The figure shows three views and two pictorial views of one solid part (mm, origin at its lowest corner). Answer the questions. Coordinates: 2 decimals unless noted, no trailing zeros. Write each loop counter-clockwise with the first axis right and the second up, starting at its lowest first coordinate (ties: lowest second). Pieces come first, ordered by that corner, then holes.
Item 1: Straight lines are drawn through the part: probe 1 along Y at (x, z) = (12.75, 141.5) (1 decimal); probe 2 along X at (y, z) = (15.5, 110); probe 3 along X at (y, z) = (5.5, 56.5) (1 decimal). For each, find the intervals that lie inside material, in ascending order.
Item 2: Section C-C (y = 18.5) is taken. Give the vertices of the cut face in (x, z) (1 decimal).
Item 3: Each of these flat-tipped pins is pushed along its axis until it touches: P1, Ø8, axis at x = 4, z = 95.5, coming from the -Y side; P2, Ø10, axis at y = 29.5, z = 152.5, coming from the +X side; P3, Ø3, axis at x = 1.5, z = 200, coming from the -Y side (1 decimal); P4, Ø1.9, axis at x = 4, z = 201.5, coming from the +Y side (1 decimal). Where does it stop, or does it pass through?
Item 4: Determine the mould class of the marked faces 1, 2, 3 and 4 for opening direction Y: released by +Y, released by -Y, zero draft, split by the parting line, or undercut.
Item 5: Section A-A (x = 10.5) is taken. Give the vertices of the cut face in (y, z) (1 decimal), then the cut area to 3 significant figures.
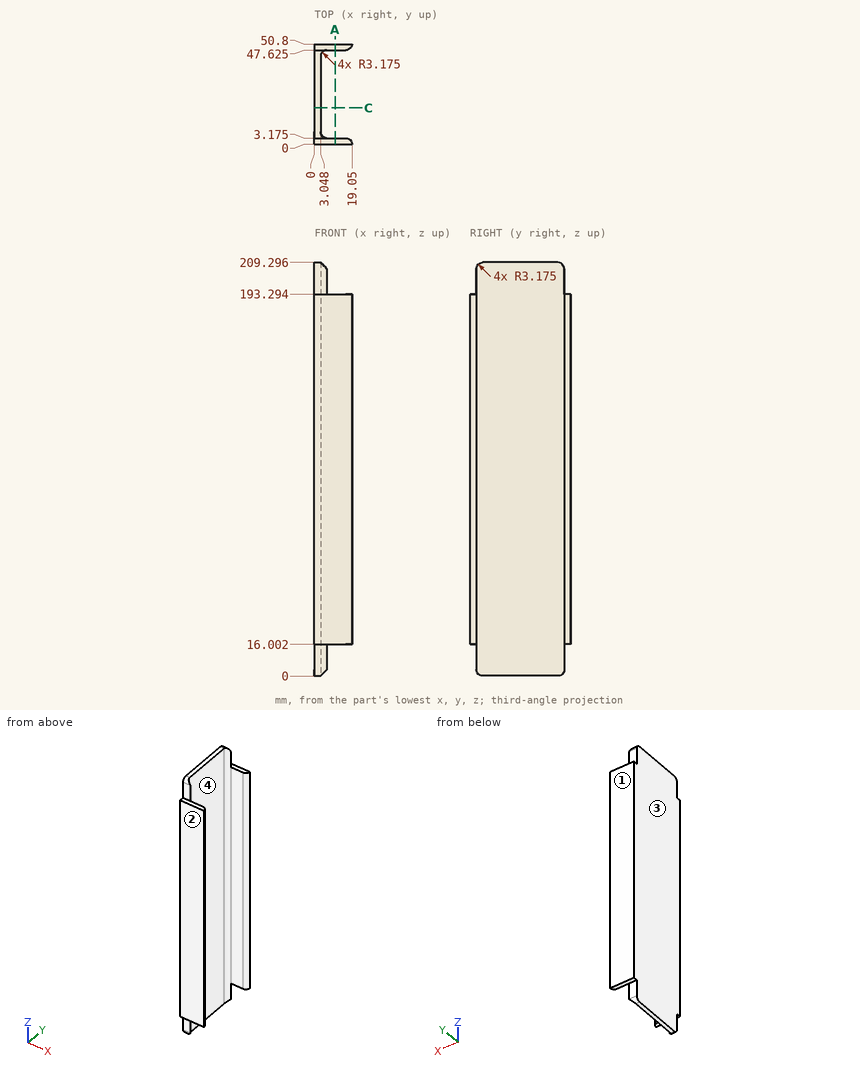
Established:
1. probe 1: y = 0 to 3.2, 47.6 to 50.8
1. probe 2: x = 0 to 3.05
1. probe 3: x = 0 to 3.2
2. outline: (0, 0) - (3, 0) - (3, 209.3) - (0, 209.3) - close
3. P1: stops at y = 0
3. P2: stops at x = 3.05
3. P3: stops at y = 3.2
3. P4: stops at y = 47.6
4. face 1: released by +Y
4. face 2: released by -Y
4. face 3: zero draft
4. face 4: undercut
5. outline: (0, 16) - (3.2, 16) - (3.2, 193.3) - (0, 193.3) - close; (47.6, 16) - (50.8, 16) - (50.8, 193.3) - (47.6, 193.3) - close
5. area: 1,130 mm2
